Verification items for the finished model (mm, model axes). A direction names the side the tool comes from. Round coordinates to 2 decimals unless told otherwise and drop trailing zeros. Order: outer loops, then holes, each group sorted by start corner. A loop starts at its lowest first (then second) coordinate and runs counter-clockwise, first axis right, second up. Notation, with made-up numbers: M -25.5,46.25 L -18.5,46.25 A8 cw -18.5,61.25 Z; hole C 65.25,30 d10. An arc over 180 degrees is marked long. Use one line per item in the form item = value. Start each with the question number.
Item 1: Go/stop test with flat-tipped pins: pin 1 Ø6 at (y, z) = (-3.5, 5.5) entering from -X; pin 2 Ø6 at (x, y) = (0, 0) entering from -Z; pin 3 Ø3 at (x, z) = (3.5, -3.5) entering from +Y; pin 4 Ø3 at (x, z) = (-3, -0.5) entering from -Y. Record where each tip stops, or that it passes through.
Item 2: Thickness scan on probe 1 along Z at (x, y) = (-3.5, -4.75); probe 2 along Y at (x, z) = (0, -8.7); probe 3 along Y at (x, z) = (-0.5, -4.5). Record the ranges inside material, lowest first. Write a range as [from, to].
Item 3: Cross-section at A-A on x = 0.5. Enter the section's corners in (y, z), then the cut area to 3 significant figures.
Item 4: Tool access check on faces 4 (the cylindrical face through (-4.83, 1.29, -0.91)), 5 (the cylindrical face through (-4.98, -0.44, -0.91)), 6 (the flat face through (1.4, 4.5, -7.5)), 7 (the cylindrical face through (1.3, -4.83, -0.91)). Record the directions out of +Z, -Z, +X, -X, +Y, -Y that give a thin tool (end or side, any length) a straight path to the whole face; none if there is none.
Item 5: Release check for a two-part mould opening along Z. For faces 1 (the flat face through (-3, -4, 5.5)), 2 (the cylindrical face through (6, 0, -8)), 3 (the flat face through (3, 0, 7.5)) record: +Z half, -Z half, draft (parallel to the pull), parting line (faces both ways), or undercut.
from build123d import *

# Parameters (mm, degrees)
CROQUIS1_R                   = 2.5
SALIENTE_EXTRUIR1_DEPTH      = 7.5
SALIENTE_EXTRUIR1_DEPTH_BACK = 7.5
CROQUIS2_R                   = 6
CROQUIS2_R_2                 = 2.5
SALIENTE_EXTRUIR2_DEPTH      = 2
CROQUIS3_R                   = 6
CROQUIS3_R_2                 = 2.5
SALIENTE_EXTRUIR3_DEPTH      = 2


with BuildPart() as part:
    # Croquis1 → Saliente-Extruir1 (new body, two sides)
    with BuildSketch(Plane.XY) as saliente_extruir1_sk:
        with BuildLine():
            Line((0, 4.41631546), (0, 5))
            ThreePointArc((0, 5), (0.435778714, 4.98097349), (0.868240888, 4.924038765))
            Line((0.868240888, 4.924038765), (0.766885132, 4.349221705))
            ThreePointArc((0.766885132, 4.349221705), (1.14302655, 4.26583316), (1.510468847, 4.149979049))
            Line((1.510468847, 4.149979049), (1.710100717, 4.698463104))
            ThreePointArc((1.710100717, 4.698463104), (2.113091309, 4.531538935), (2.5, 4.330127019))
            Line((2.5, 4.330127019), (2.20815773, 3.824641379))
            ThreePointArc((2.20815773, 3.824641379), (2.533094483, 3.617633837), (2.838752858, 3.383093917))
            Line((2.838752858, 3.383093917), (3.213938048, 3.830222216))
            ThreePointArc((3.213938048, 3.830222216), (3.535533906, 3.535533906), (3.830222216, 3.213938048))
            Line((3.830222216, 3.213938048), (3.383093917, 2.838752858))
            ThreePointArc((3.383093917, 2.838752858), (3.617633837, 2.533094483), (3.824641379, 2.20815773))
            Line((3.824641379, 2.20815773), (4.330127019, 2.5))
            ThreePointArc((4.330127019, 2.5), (4.531538935, 2.113091309), (4.698463104, 1.710100717))
            Line((4.698463104, 1.710100717), (4.149979049, 1.510468847))
            ThreePointArc((4.149979049, 1.510468847), (4.26583316, 1.14302655), (4.349221705, 0.766885132))
            Line((4.349221705, 0.766885132), (4.924038765, 0.868240888))
            ThreePointArc((4.924038765, 0.868240888), (4.98097349, 0.435778714), (5, 0))
            Line((5, 0), (4.41631546, 0))
            ThreePointArc((4.41631546, 0), (4.399510046, -0.384907254), (4.349221705, -0.766885132))
            Line((4.349221705, -0.766885132), (4.924038765, -0.868240888))
            ThreePointArc((4.924038765, -0.868240888), (4.829629131, -1.294095226), (4.698463104, -1.710100717))
            Line((4.698463104, -1.710100717), (4.149979049, -1.510468847))
            ThreePointArc((4.149979049, -1.510468847), (4.002541091, -1.866415563), (3.824641379, -2.20815773))
            Line((3.824641379, -2.20815773), (4.330127019, -2.5))
            ThreePointArc((4.330127019, -2.5), (4.095760221, -2.867882182), (3.830222216, -3.213938048))
            Line((3.830222216, -3.213938048), (3.383093917, -2.838752858))
            ThreePointArc((3.383093917, -2.838752858), (3.122806609, -3.122806609), (2.838752858, -3.383093917))
            Line((2.838752858, -3.383093917), (3.213938048, -3.830222216))
            ThreePointArc((3.213938048, -3.830222216), (2.867882182, -4.095760221), (2.5, -4.330127019))
            Line((2.5, -4.330127019), (2.20815773, -3.824641379))
            ThreePointArc((2.20815773, -3.824641379), (1.866415563, -4.002541091), (1.510468847, -4.149979049))
            Line((1.510468847, -4.149979049), (1.710100717, -4.698463104))
            ThreePointArc((1.710100717, -4.698463104), (1.294095226, -4.829629131), (0.868240888, -4.924038765))
            Line((0.868240888, -4.924038765), (0.766885132, -4.349221705))
            ThreePointArc((0.766885132, -4.349221705), (0.384907254, -4.399510046), (0, -4.41631546))
            Line((0, -4.41631546), (0, -5))
            ThreePointArc((0, -5), (-0.435778714, -4.98097349), (-0.868240888, -4.924038765))
            Line((-0.868240888, -4.924038765), (-0.766885132, -4.349221705))
            ThreePointArc((-0.766885132, -4.349221705), (-1.14302655, -4.26583316), (-1.510468847, -4.149979049))
            Line((-1.510468847, -4.149979049), (-1.710100717, -4.698463104))
            ThreePointArc((-1.710100717, -4.698463104), (-2.113091309, -4.531538935), (-2.5, -4.330127019))
            Line((-2.5, -4.330127019), (-2.20815773, -3.824641379))
            ThreePointArc((-2.20815773, -3.824641379), (-2.533094483, -3.617633837), (-2.838752858, -3.383093917))
            Line((-2.838752858, -3.383093917), (-3.213938048, -3.830222216))
            ThreePointArc((-3.213938048, -3.830222216), (-3.535533906, -3.535533906), (-3.830222216, -3.213938048))
            Line((-3.830222216, -3.213938048), (-3.383093917, -2.838752858))
            ThreePointArc((-3.383093917, -2.838752858), (-3.617633837, -2.533094483), (-3.824641379, -2.20815773))
            Line((-3.824641379, -2.20815773), (-4.330127019, -2.5))
            ThreePointArc((-4.330127019, -2.5), (-4.531538935, -2.113091309), (-4.698463104, -1.710100717))
            Line((-4.698463104, -1.710100717), (-4.149979049, -1.510468847))
            ThreePointArc((-4.149979049, -1.510468847), (-4.26583316, -1.14302655), (-4.349221705, -0.766885132))
            Line((-4.349221705, -0.766885132), (-4.924038765, -0.868240888))
            ThreePointArc((-4.924038765, -0.868240888), (-4.98097349, -0.435778714), (-5, 0))
            Line((-5, 0), (-4.41631546, 0))
            ThreePointArc((-4.41631546, 0), (-4.399510046, 0.384907254), (-4.349221705, 0.766885132))
            Line((-4.349221705, 0.766885132), (-4.924038765, 0.868240888))
            ThreePointArc((-4.924038765, 0.868240888), (-4.829629131, 1.294095226), (-4.698463104, 1.710100717))
            Line((-4.698463104, 1.710100717), (-4.149979049, 1.510468847))
            ThreePointArc((-4.149979049, 1.510468847), (-4.002541091, 1.866415563), (-3.824641379, 2.20815773))
            Line((-3.824641379, 2.20815773), (-4.330127019, 2.5))
            ThreePointArc((-4.330127019, 2.5), (-4.095760221, 2.867882182), (-3.830222216, 3.213938048))
            Line((-3.830222216, 3.213938048), (-3.383093917, 2.838752858))
            ThreePointArc((-3.383093917, 2.838752858), (-3.122806609, 3.122806609), (-2.838752858, 3.383093917))
            Line((-2.838752858, 3.383093917), (-3.213938048, 3.830222216))
            ThreePointArc((-3.213938048, 3.830222216), (-2.867882182, 4.095760221), (-2.5, 4.330127019))
            Line((-2.5, 4.330127019), (-2.20815773, 3.824641379))
            ThreePointArc((-2.20815773, 3.824641379), (-1.866415563, 4.002541091), (-1.510468847, 4.149979049))
            Line((-1.510468847, 4.149979049), (-1.710100717, 4.698463104))
            ThreePointArc((-1.710100717, 4.698463104), (-1.294095226, 4.829629131), (-0.868240888, 4.924038765))
            Line((-0.868240888, 4.924038765), (-0.766885132, 4.349221705))
            ThreePointArc((-0.766885132, 4.349221705), (-0.384907254, 4.399510046), (0, 4.41631546))
        make_face()
        Circle(CROQUIS1_R, mode=Mode.SUBTRACT)
    extrude(amount=SALIENTE_EXTRUIR1_DEPTH)
    extrude(saliente_extruir1_sk.sketch, amount=-SALIENTE_EXTRUIR1_DEPTH_BACK)

    # Croquis2 → Saliente-Extruir2 (add)
    with BuildSketch(Plane.XY.offset(7.5)):
        Circle(CROQUIS2_R)
        Circle(CROQUIS2_R_2, mode=Mode.SUBTRACT)
    extrude(amount=-SALIENTE_EXTRUIR2_DEPTH)

    # Croquis3 → Saliente-Extruir3 (add)
    with BuildSketch(Plane(origin=(0, 0, -7.5), x_dir=(-1, 0, 0), z_dir=(0, 0, -1))):
        Circle(CROQUIS3_R)
        Circle(CROQUIS3_R_2, mode=Mode.SUBTRACT)
    extrude(amount=SALIENTE_EXTRUIR3_DEPTH)


solid = part.part
Output values:
q1.pin_1 = -5.98
q1.pin_2 = -9.5
q1.pin_3 = 4.58
q1.pin_4 = -4.7
q2.probe_1 = [-9.5, -7.5], [5.5, 7.5]
q2.probe_2 = [-6, -2.5], [2.5, 6]
q2.probe_3 = [-4.97, -2.45], [2.45, 4.39]
q3.outline = M -5.98,-9.5 L -2.45,-9.5 L -2.45,7.5 L -5.98,7.5 L -5.98,5.5 L -4.39,5.5 L -4.39,-7.5 L -5.98,-7.5 Z; M 2.45,-9.5 L 5.98,-9.5 L 5.98,-7.5 L 4.97,-7.5 L 4.97,5.5 L 5.98,5.5 L 5.98,7.5 L 2.45,7.5 Z
q3.area = 86.3 mm2
q4.face_4 = -X, +Y
q4.face_5 = -X, -Y
q4.face_6 = none
q4.face_7 = +X, -Y
q5.face_1 = undercut
q5.face_2 = draft
q5.face_3 = +Z half
